Design review of the part built by this model. Coordinates are the model's own, in mm. A direction names the side the tool comes from. Give positions to 0.01 mm unless a question says otherwise; leave off trailing zeros. Loops run counter-clockwise (first coordinate to the right, second up) from the corner with the lowest first, then second, coordinate; pieces in that order, holes last. Notation, with made-up numbers: (-11.5, -38.75) -> (6.5, -38.75) arc R34 cw to (6.5, -4.75) -> close; hole circle Ø11 at (47.25, 55.25). An arc over 180 degrees is marked (long way). Use a Markdown table: item, result. Add a question column.
1. For pin 1 Ø6 at (x, z) = (25, 0) entering from +Y; pin 2 Ø1.5 at (y, z) = (5.5, -1) entering from -X; pin 3 Ø3 at (x, y) = (1, 5.5) entering from +Z, all flat-tipped, find the tip position at first contact; note any pin that passes through.
2. Add section C-C (y = 2). State the section outline as (x, z) points.
3. For faces 1 (the flat face through (0, 3.35, -19)), 2 (the flat face through (11, 6.35, 6)), list the 3-axis set-ups (+Z, -Z, +X, -X, +Y, -Y) from which the entire face can be reached by the end or side of a thin tool; tool diameter is ignored.
4. Add section D-D (z = 27). State the section outline as (x, y) points, and give its area (3 significant figures).
5. To check wall thickness, follow line 1 (Z direction, x = 0.5, y = 3.5); line 2 (X direction, y = 6, z = 1.5); line 3 (Z direction, x = 0, y = 2.25). State the ranges of each line that lie inside material, in increasing order.
6. Add section A-A (x = 0). State the section outline as (y, z) points.
7. Add section B-B (z = 0). State the section outline as (x, y) points.
8. Draft analysis for pull direction Z (two halves, no side actions). For faces 3 (the cylindrical face through (0.31, 4.87, -17.21)), 4 (the flat face through (9, 0, 9)), state which applies: pulls with the +Z half, pulls with the -Z half, needs draft (parallel to the pull), parting line crosses it, or undercut.
Solid Edge part; units mm, degrees
sketch "Sketch1" plane through (0, 0, 0) normal (0, -1, 0) x (1, 0, 0)
  circle A0 centre (0, 0) radius 37.211
  circle A1 centre (0, 0) radius 12.25
extrude "Protrusion1" add sketch "Sketch1" against normal blind 6.35
extrude "Cutout1" [suppressed]
pattern "Pattern1" [suppressed]
hole "Hole_1" at (25, 0, 0) direction (0, 1, 0) diameter 5.2197 end up to next
hole "Hole1" at (-25, 0, 0) direction (0, 1, 0) diameter 5.2197 end up to next
sketch "Sketch2" plane through (0, 6.35, 0) normal (0, 1, 0) x (-1, 0, 0)
  line L0 (25, -5.4993) -> (29.7625, -2.7496)
  line L1 (29.7625, -2.7496) -> (29.7625, 2.7496)
  line L2 (29.7625, 2.7496) -> (25, 5.4993)
  line L3 (25, 5.4993) -> (20.2375, 2.7496)
  line L4 (20.2375, 2.7496) -> (20.2375, -2.7496)
  line L5 (20.2375, -2.7496) -> (25, -5.4993)
  line L6 (-25, -5.4993) -> (-20.2375, -2.7496)
  line L7 (-20.2375, -2.7496) -> (-20.2375, 2.7496)
  line L8 (-20.2375, 2.7496) -> (-25, 5.4993)
  line L9 (-25, 5.4993) -> (-29.7625, 2.7496)
  line L10 (-29.7625, 2.7496) -> (-29.7625, -2.7496)
  line L11 (-29.7625, -2.7496) -> (-25, -5.4993)
extrude "ExtrudedCutout_2" cut sketch "Sketch2" against normal blind 3
sketch "Sketch3" plane through (0, 6.35, 0) normal (0, 1, 0) x (-1, 0, 0)
  arc A0 (-30.2684, 11.0168) -> (30.2684, 11.0168) centre (0, 0) cw
  line L0 (16.173, 5.8865) -> (30.2684, 11.0168)
  line L1 (-16.1835, 5.8579) -> (-30.2684, 11.0168)
  arc A1 (-16.1834, 5.8579) -> (16.173, 5.8865) centre (0, 0) cw
  line L2 (-16.1835, -5.8579) -> (-30.2684, -11.0168)
  line L3 (16.173, -5.8865) -> (30.2684, -11.0168)
  arc A2 (16.173, -5.8865) -> (-16.1835, -5.8579) centre (0, 0) cw
  arc A3 (30.2684, -11.0168) -> (-30.2684, -11.0168) centre (0, 0) cw
extrude "ExtrudedCutout_3" cut sketch "Sketch3" against normal blind 3
Taken from the geometry:
| question | item | result |
|---|---|---|
| 1 | pin 1 | stops at y = 3.35 |
| 1 | pin 2 | stops at x = -37.21 |
| 1 | pin 3 | stops at z = 37.21 |
| 2 | outline | circle Ø74.42 at (0, 0); hole circle Ø5.22 at (-25, 0); hole circle Ø24.5 at (0, 0); hole circle Ø5.22 at (25, 0) |
| 3 | face 1 | +Y |
| 3 | face 2 | +Z, -Z, +X, -X, +Y |
| 4 | outline | (-25.61, 0) -> (25.61, 0) -> (25.61, 6.35) -> (17.57, 6.35) -> (17.57, 3.35) -> (-17.57, 3.35) -> (-17.57, 6.35) -> (-25.61, 6.35) -> close |
| 4 | area | 220 mm^2 |
| 5 | line 1 | z = -37.21 to -32.21, -17.2 to -12.24, 12.24 to 17.2, 32.21 to 37.21 |
| 5 | line 2 | x = -37.18 to -29.76, -20.24 to -12.16, 12.16 to 20.24, 29.76 to 37.18 |
| 5 | line 3 | z = -37.21 to -12.25, 12.25 to 37.21 |
| 6 | outline | (0, -37.21) -> (6.35, -37.21) -> (6.35, -32.21) -> (3.35, -32.21) -> (3.35, -17.21) -> (6.35, -17.21) -> (6.35, -12.25) -> (0, -12.25) -> close; (0, 12.25) -> (6.35, 12.25) -> (6.35, 17.21) -> (3.35, 17.21) -> (3.35, 32.21) -> (6.35, 32.21) -> (6.35, 37.21) -> (0, 37.21) -> close |
| 7 | outline | (-37.21, 0) -> (-27.61, 0) -> (-27.61, 3.35) -> (-29.76, 3.35) -> (-29.76, 6.35) -> (-37.21, 6.35) -> close; (-22.39, 0) -> (-12.25, 0) -> (-12.25, 6.35) -> (-20.24, 6.35) -> (-20.24, 3.35) -> (-22.39, 3.35) -> close; (12.25, 0) -> (22.39, 0) -> (22.39, 3.35) -> (20.24, 3.35) -> (20.24, 6.35) -> (12.25, 6.35) -> close; (27.61, 0) -> (37.21, 0) -> (37.21, 6.35) -> (29.76, 6.35) -> (29.76, 3.35) -> (27.61, 3.35) -> close |
| 8 | face 3 | undercut |
| 8 | face 4 | needs draft |
